CAD build for the part. Positions are in the model's coordinates, mm. A direction names the side the tool comes from. Round coordinates to 2 decimals unless told otherwise and drop trailing zeros. Loops run counter-clockwise (first coordinate to the right, second up) from the corner with the lowest first, then second, coordinate; pieces in that order, holes last. Notation, with made-up numbers: (-9.5, 42.25) - (40.5, 42.25) arc R16 ccw to (40.5, 52.25) - close; hole circle Ø2 at (40, -23). An arc over 180 degrees is marked (long way). One line per question, with ' | ' between items.
```python
from build123d import *

# Parameters (mm, degrees)
F0_W     = 2280
F0_H     = 950
F1_DEPTH = 400
F2_W     = 179.1080534458
F2_H     = 773.6296027899
F2_H_2   = 176.3703972101
F2_W_2   = 1947.9051530361
F2_W_3   = 152.9867935181
F3_DEPTH = 238.83933


with BuildPart() as f1:
    # F0 (on Front) → F1 (new body)
    with BuildSketch(Plane.XZ):
        with Locations((1140, 475)):
            Rectangle(F0_W, F0_H)
    extrude(amount=F1_DEPTH)

    # F2 (on face) → F3 (join)
    with BuildSketch(Plane.XZ.offset(400)):
        with Locations((89.5540267229, 563.1851986051)):
            Rectangle(F2_W, F2_H)
        with Locations((89.5540267229, 88.1851986051)):
            Rectangle(F2_W, F2_H_2)
        with Locations((1153.0606299639, 88.1851986051)):
            Rectangle(F2_W_2, F2_H_2)
        with Locations((2203.506603241, 88.1851986051)):
            Rectangle(F2_W_3, F2_H_2)
        with Locations((2203.506603241, 563.1851986051)):
            Rectangle(F2_W_3, F2_H)
    extrude(amount=F3_DEPTH)


solid = f1.part
```
(1) Cut at A-A, the plane y = -480. Write the cut outline in (x, z), then the cut area to 3 significant figures.
Results found:
outline: (0, 0) - (2280, 0) - (2280, 950) - (2127.01, 950) - (2127.01, 176.37) - (179.11, 176.37) - (179.11, 950) - (0, 950) - close | area: 659,000 mm²
(2) Drop a flat-ended pin along its axis: P1, Ø1, axis at x = 1177, z = 479, coming from the -Y side. Give the stop position or say it passes through.
Results found:
P1: stops at y = -400
(3) Cut at B-B, the plane z = 854.5. Write the cut outline in (x, y), then the cut area to 3 significant figures.
Results found:
outline: (0, -638.84) - (179.11, -638.84) - (179.11, -400) - (2127.01, -400) - (2127.01, -638.84) - (2280, -638.84) - (2280, 0) - (0, 0) - close | area: 991,000 mm²
(4) Tool access for faces 1 (the face through (1124, 0, 482)), 2 (the face through (1139, -400, 569)): list every direction of +Z, -Z, +X, -X, +Y, -Y with a clear straight run to the whole face (end or side of a thin tool).
Results found:
face 1: +Z, -Z, +X, -X, +Y | face 2: +Z, -Y
(5) Probe L1, parallel to X at y = -605.5, z = 509.5; L2, parallel to Z at x = 1602, y = -595.5; L3, parallel to Y at x = 539, z = 737. List the from-to ranges inside material, lowest first.
Results found:
L1: x = 0 to 179.11, 2127.01 to 2280 | L2: z = 0 to 176.37 | L3: y = -400 to 0
(6) Cut at C-C, the plane x = 1529. Write the cut outline in (y, z), then the cut area to 3 significant figures.
Results found:
outline: (-638.84, 0) - (0, 0) - (0, 950) - (-400, 950) - (-400, 176.37) - (-638.84, 176.37) - close | area: 422,000 mm²
(7) Two-plate mould, pull along X, no slides. Class faces 3 (the face through (2127.013, -518, 558)), 4 (the face through (1124, -244, 950)), 5 (the face through (0, -315, 482)), 6 (the face through (1167, -518, 176.37)): released by +X, released by -X, zero draft, split by the parting line, or undercut.
Results found:
face 3: undercut | face 4: zero draft | face 5: released by -X | face 6: undercut
